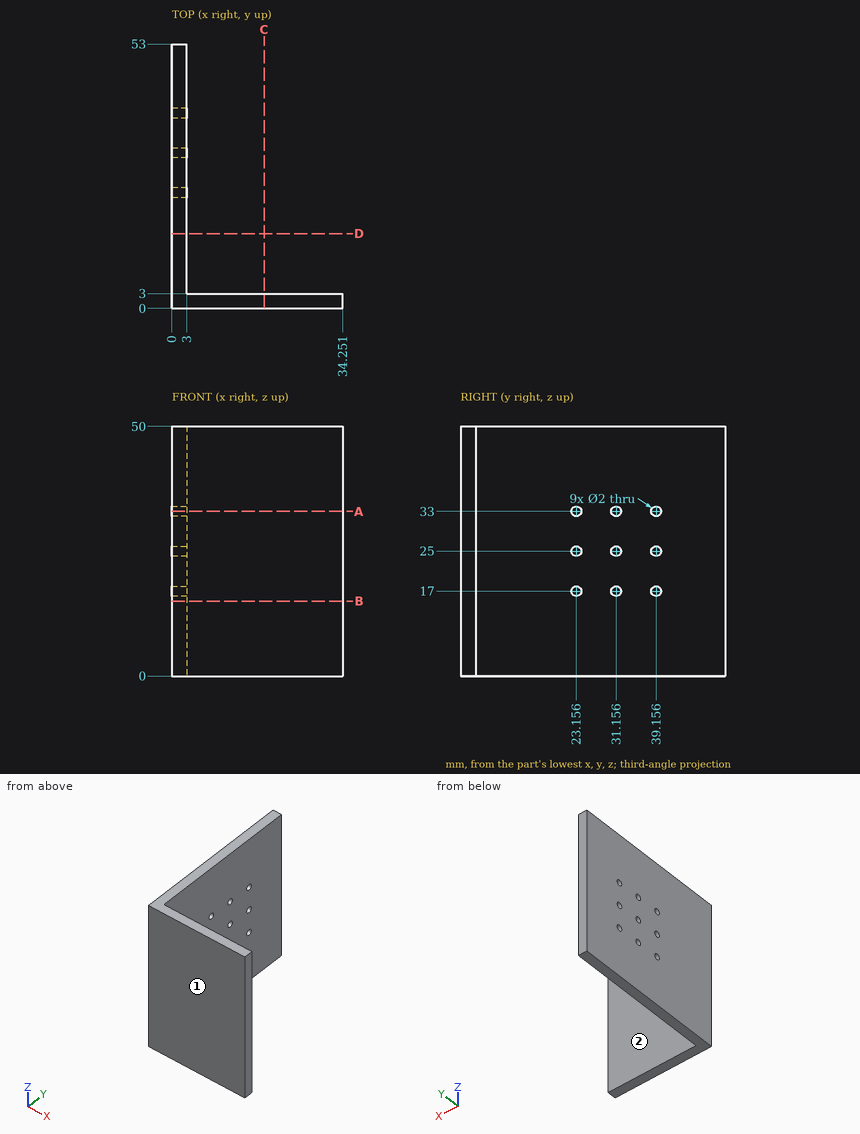
Can you work these out from the drawing? Everything is in mm from the part's minimum corner. A direction names the side the tool comes from. Round coordinates to 2 decimals unless told otherwise and drop trailing zeros. Loops run counter-clockwise (first coordinate to the right, second up) from the corner with the lowest first, then second, coordinate; pieces in that order, holes last. Notation, with made-up numbers: M -28.5,-22 L -5.5,-22 A12 cw -5.5,-5 Z; hole C 13.5,-15.75 d11. An arc over 180 degrees is marked long. Write item = value, one per line.
1. Will these pins go through, and if not, where does the flat tip stop? P1, Ø8, axis at y = 36, z = 27.5, coming from the +X side; P2, Ø9.5, axis at x = 11, z = 36.5, coming from the +Y side.
Results below:
P1 = 3
P2 = 3
2. I want a section at A-A, the plane z = 33. Write out the boundary of the cut face in (x, y).
Results below:
outline = M 0,0 L 34.25,0 L 34.25,3 L 3,3 L 3,22.16 L 0,22.16 Z; M 0,24.16 L 3,24.16 L 3,30.16 L 0,30.16 Z; M 0,32.16 L 3,32.16 L 3,38.16 L 0,38.16 Z; M 0,40.16 L 3,40.16 L 3,53 L 0,53 Z
3. I need wall thicknesses on probe 1 along Y at (x, z) = (1.25, 17); probe 2 along X at (y, z) = (20.5, 11). Which ranges of each line are inside material? Lowest first, please.
Results below:
probe_1 = 0 to 22.16, 24.16 to 30.16, 32.16 to 38.16, 40.16 to 53
probe_2 = 0 to 3
4. I want a section at C-C, the plane x = 18.5. Write out the boundary of the cut face in (y, z).
Results below:
outline = M 0,0 L 3,0 L 3,50 L 0,50 Z
5. I want a section at B-B, the plane z = 15. Write out the boundary of the cut face in (x, y), and give its area (3 significant figures).
Results below:
outline = M 0,0 L 34.25,0 L 34.25,3 L 3,3 L 3,53 L 0,53 Z
area = 253 mm²
6. Which directions (+Z, -Z, +X, -X, +Y, -Y) give clear straight access to the entire face, cutting with the end or side of a thin tool? Please do the marked faces 1 and 2.
Results below:
face_1 = +Z, -Z, +X, -X, -Y
face_2 = +Z, -Z, +X, +Y
